from build123d import *

# Parameters (mm, degrees)
SKETCH1_R           = 1.125
BOSS_EXTRUDE1_DEPTH = 3.2
SKETCH2_W           = 3.3
SKETCH2_H           = 4.8
CUT_EXTRUDE1_DEPTH  = 8.9
SKETCH4_R           = 2.4
CUT_EXTRUDE2_DEPTH  = 5


with BuildPart() as part:
    # Sketch1 → Boss-Extrude1 (new body, symmetric)
    with BuildSketch(Plane.XY):
        with BuildLine():
            Line((-3.5, 0), (-3.5, -11.2))
            Line((-3.5, -11.2), (4.3, -11.2))
            Line((4.3, -11.2), (4.3, -8))
            Line((4.3, -8), (2.1, -8))
            Line((2.1, -8), (2.1, -2.8))
            ThreePointArc((2.1, -2.8), (1.565247584, 3.130495168), (-3.5, 0))
        make_face()
        Circle(SKETCH1_R, mode=Mode.SUBTRACT)
    extrude(amount=BOSS_EXTRUDE1_DEPTH, both=True)

    # Sketch2 → Cut-Extrude1 (cut)
    with BuildSketch(Plane.XZ.offset(11.2)):
        with Locations((-0.45, 0)):
            Rectangle(SKETCH2_W, SKETCH2_H)
    extrude(amount=-CUT_EXTRUDE1_DEPTH, mode=Mode.SUBTRACT)

    # Sketch4 → Cut-Extrude2 (cut)
    with BuildSketch(Plane.ZY.offset(3.5)):
        with Locations((0, 0.5)):
            Circle(SKETCH4_R)
    extrude(amount=-CUT_EXTRUDE2_DEPTH, mode=Mode.SUBTRACT)


solid = part.part
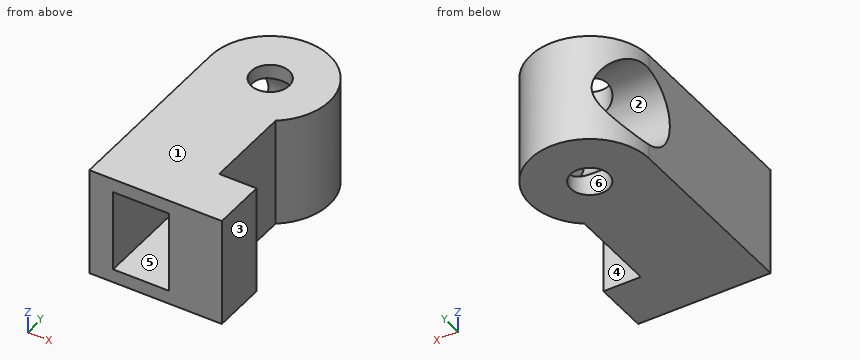
Design review of the part built by this model. Coordinates are the model's own, in mm. Face numbers are marked on the shaded views. A direction names the side the tool comes from. Round coordinates to 2 decimals unless told otherwise and drop trailing zeros. Write each loop counter-clockwise with the first axis right and the second up, starting at its lowest first coordinate (ties: lowest second). Pieces come first, ordered by that corner, then holes.
Item 1: Consider section C-C on y = 0.5. Give the boundary of the cut face in (x, z), and give its area (3 significant figures).
Item 2: For the marked faces 4, 5 and 6, list the 3-axis set-ups (+Z, -Z, +X, -X, +Y, -Y) from which the entire face can be reached by the end or side of a thin tool; tool diameter is ignored.
Item 3: Consider section A-A on y = -4. Give the boundary of the cut face in (x, z).
Item 4: Wall thickness on L1, parallel to X at y = -3, z = -0.25; L2, parallel to X at y = -9.5, z = 1.5; L3, parallel to Y at x = 0, z = 2.85 (3 decimals): over which ranges is each line inside the solid? List them lowest first.
Item 5: Consider section B-B on x = 0. Give the boundary of the cut face in (y, z) (3 decimals), and give its area (3 significant figures).
Item 6: For pin 1 Ø0.7 at (x, z) = (3.5, 1) entering from +Y; pin 2 Ø1.5 at (x, z) = (3, -1.5) entering from +Y, all flat-tipped, find the tip position at first contact; note any pin that passes through.
Item 7: Draft analysis for pull direction Z (two halves, no side actions). For the marked faces 1, 2 and 3, state which applies: released by +Z, released by -Z, zero draft, split by the parting line, or undercut.
Item 8: Consider section D-D on z = 1.5. Give the boundary of the cut face in (x, y), and give its area (3 significant figures).
Check values:
1. outline: (-3.46, -3.2) - (-1.01, -3.2) - (-1.01, -2.4) - (-3.46, -2.4) - close; (-3.46, 2.4) - (-1.01, 2.4) - (-1.01, 3.2) - (-3.46, 3.2) - close; (1.01, -3.2) - (3.46, -3.2) - (3.46, 3.2) - (1.01, 3.2) - (1.01, 2.4) - (1.5, 2.4) - (1.5, -2.4) - (1.01, -2.4) - close
1. area: 17.3 mm2
2. face 4: +Z, -Z, +X
2. face 5: -Y
2. face 6: +Z, -Z
3. outline: (-3.5, -3.2) - (2.1, -3.2) - (2.1, 3.2) - (-3.5, 3.2) - close; hole (-2.1, -2.4) - (1.2, -2.4) - (1.2, 2.4) - (-2.1, 2.4) - close
4. L1: x = -3.5 to -2.1, 1.2 to 2.1
4. L2: x = -3.5 to -2.1, 1.2 to 4.3
4. L3: y = -11.2 to -1.125, 1.125 to 3.5
5. outline: (-11.2, -3.2) - (-1.125, -3.2) - (-1.125, -1.766) arc R2.4 cw to (-1.125, 1.766) - (-1.125, 3.2) - (-11.2, 3.2) - (-11.2, 2.4) - (-2.3, 2.4) - (-2.3, -2.4) - (-11.2, -2.4) - close; (1.125, -3.2) - (3.5, -3.2) - (3.5, 3.2) - (1.125, 3.2) - (1.125, 2.317) arc R2.4 cw to (1.125, -2.317) - close
5. area: 29.0 mm2
6. pin 1: stops at y = 1.53
6. pin 2: stops at y = 2.68
7. face 1: released by +Z
7. face 2: undercut
7. face 3: zero draft
8. outline: (-3.5, -11.2) - (-2.1, -11.2) - (-2.1, -2.3) - (1.2, -2.3) - (1.2, -11.2) - (4.3, -11.2) - (4.3, -8) - (2.1, -8) - (2.1, -2.8) arc R3.5 ccw (long way) to (-2.57, 2.37) - (1.5, 2.37) - (1.5, -1.37) - (-3.5, -1.37) - close
8. area: 44.3 mm2
